Read the model definition and answer for the solid it produces. Units are mm, in the model's axes. A direction names the side the tool comes from. Give positions to 0.01 mm unless a question says otherwise; leave off trailing zeros. Write each loop counter-clockwise with the first axis right and the second up, starting at its lowest first coordinate (ties: lowest second). Pieces come first, ordered by that corner, then holes. Notation, with made-up numbers: M -18.5,57.25 L 35.5,57.25 A24 ccw 35.5,87.25 Z; hole C 42.5,-8 d5. An arc over 180 degrees is marked long. Answer as CSV lines item,"result". Start each with the question number.
```python
from build123d import *

# Parameters (mm, degrees)
T_LE_DE_BASE_PLI_E1_DEPTH             = 20.5
ESQUISSE8_W                           = 24
ESQUISSE8_H                           = 2
BOSS_EXTRU_1_DEPTH                    = 8.5
T_LE_PLI_E_SUR_AR_TE1_STRIP_W         = 10
T_LE_PLI_E_SUR_AR_TE1_STRIP_H         = 2
T_LE_PLI_E_SUR_AR_TE1_STRIP_CUT_DEPTH = 8.5
T_LE_PLI_E_SUR_AR_TE1_DEPTH           = 8.5
ESQUISSE12_W                          = 1.5
ESQUISSE12_H                          = 12
ENL_V_MAT_EXTRU_1_DEPTH               = 8.5
DIAM_TRE_DU_PER_AGE_4_0_4_1_D         = 4
DIAM_TRE_DU_PER_AGE_8_0_8_1_D         = 8
F_3_0_3_DIAMETER_HOLE3_D              = 3
R_P_TITION_CIRCULAIRE1_COUNT          = 4
DIAM_TRE_DU_PER_AGE_4_0_4_2_D         = 4
F_3_0_3_DIAMETER_HOLE1_D              = 3
CIRPATTERN1_COUNT                     = 4
CONG_1_R                              = 4
DIAM_TRE_DU_PER_AGE_8_0_8_2_D         = 8
F_3_0_3_DIAMETER_HOLE2_D              = 3
R_P_TITION_CIRCULAIRE2_COUNT          = 4


# Sheet-metal steps are written as plain solids
with BuildPart() as part:
    # Esquisse1 → Tôle de base pliée1 (new body)
    with BuildSketch(Plane(origin=(0, 0, 0), x_dir=(0, 0, -1), z_dir=(1, 0, 0))):
        with BuildLine():
            Line((0, 27), (0, 3))
            ThreePointArc((0, 3), (-0.878679656, 0.878679656), (-3, 0))
            Line((-3, 0), (-37.5, 0))
            Line((-37.5, 0), (-37.5, 2))
            Line((-37.5, 2), (-3, 2))
            ThreePointArc((-3, 2), (-2.292893219, 2.292893219), (-2, 3))
            Line((-2, 3), (-2, 27))
            Line((-2, 27), (0, 27))
        make_face()
    extrude(amount=T_LE_DE_BASE_PLI_E1_DEPTH)

    # Esquisse8 → Boss.-Extru.1 (add)
    with BuildSketch(Plane(origin=(20.5, 0, 0), x_dir=(0, 0, -1), z_dir=(1, 0, 0))):
        with Locations((-19, 1)):
            Rectangle(ESQUISSE8_W, ESQUISSE8_H)
    extrude(amount=BOSS_EXTRU_1_DEPTH)

    # Tôle pliée sur arête1 strip (across the edge) → Tôle pliée sur arête1 strip cut (cut)
    with BuildSketch(Plane(origin=(20.5, 2, 31), x_dir=(0, 0, -1), z_dir=(1, 0, 0))):
        with Locations((-4, -1)):
            Rectangle(T_LE_PLI_E_SUR_AR_TE1_STRIP_W, T_LE_PLI_E_SUR_AR_TE1_STRIP_H)
    extrude(amount=T_LE_PLI_E_SUR_AR_TE1_STRIP_CUT_DEPTH, mode=Mode.SUBTRACT)

    # Tôle pliée sur arête1 section (across the edge) → Tôle pliée sur arête1 (add)
    with BuildSketch(Plane(origin=(20.5, 2, 31), x_dir=(0, 0, -1), z_dir=(1, 0, 0))):
        with BuildLine():
            Line((-2, 1), (-2, 25))
            Line((-2, 25), (0, 25))
            Line((0, 25), (0, 1))
            ThreePointArc((0, 1), (0.292893219, 0.292893219), (1, 0))
            Line((1, 0), (1, -2))
            ThreePointArc((1, -2), (-1.121320344, -1.121320344), (-2, 1))
        make_face()
    extrude(amount=T_LE_PLI_E_SUR_AR_TE1_DEPTH)

    # Esquisse12 → Enlèv. mat.-Extru.1 (cut)
    with BuildSketch(Plane(origin=(0, 2, 0), x_dir=(1, 0, 0), z_dir=(0, 1, 0))):
        with Locations((19.75, -31.5)):
            Rectangle(ESQUISSE12_W, ESQUISSE12_H)
    extrude(amount=-ENL_V_MAT_EXTRU_1_DEPTH, mode=Mode.SUBTRACT)

    # Diamètre du perçage Ø4.0 (4)1 (through all)
    with Locations(Plane(origin=(0, 2, 0), x_dir=(1, 0, 0), z_dir=(0, 1, 0))):
        with Locations((24.25, -12.13), (24.25, -22.13)):
            Hole(DIAM_TRE_DU_PER_AGE_4_0_4_1_D / 2)

    # Diamètre du perçage Ø8.0 (8)1 (through all)
    with Locations(Plane(origin=(0, 2, 0), x_dir=(1, 0, 0), z_dir=(0, 1, 0))):
        with Locations((10.75, -22.63)):
            Hole(DIAM_TRE_DU_PER_AGE_8_0_8_1_D / 2)

    # Ø3.0 (3) Diameter Hole3 (through all)
    with Locations(Plane(origin=(0, 2, 0), x_dir=(1, 0, 0), z_dir=(0, 1, 0))):
        with Locations((10.75, -15.63)):
            f_3_0_3_diameter_hole3 = Hole(F_3_0_3_DIAMETER_HOLE3_D / 2)

    # Répétition circulaire1: Ø3.0 (3) Diameter Hole3 ×4 about axis
    r_p_tition_circulaire1_axis = Axis((10.75, 0, 22.63), (0, 1, 0))
    for i in range(1, R_P_TITION_CIRCULAIRE1_COUNT):
        add(f_3_0_3_diameter_hole3.rotate(r_p_tition_circulaire1_axis, i * 360 / R_P_TITION_CIRCULAIRE1_COUNT), mode=Mode.SUBTRACT)

    # Diamètre du perçage Ø4.0 (4)2 (through all)
    with Locations(Plane.XY.offset(33)):
        with Locations((24.25, 19.87), (24.25, 9.87)):
            Hole(DIAM_TRE_DU_PER_AGE_4_0_4_2_D / 2)

    # Ø3.0 (3) Diameter Hole1 (through all)
    with Locations(Plane.XY.offset(2)):
        with Locations((11, 14.87), (11, 21.87)):
            f_3_0_3_diameter_hole1 = Hole(F_3_0_3_DIAMETER_HOLE1_D / 2)

    # CirPattern1: Ø3.0 (3) Diameter Hole1 ×4 about axis
    cirpattern1_axis = Axis((11, 14.87, 0), (0, 0, 1))
    for i in range(1, CIRPATTERN1_COUNT):
        add(f_3_0_3_diameter_hole1.rotate(cirpattern1_axis, i * 360 / CIRPATTERN1_COUNT), mode=Mode.SUBTRACT)

    # Congé1
    cong_1_edges = [part.edges().sort_by_distance(p)[0] for p in [
        (20.5, 27, 1),
        (29, 1, 7),
        (29, 27, 32),
        (19, 1, 37.5),
    ]]
    fillet(cong_1_edges, radius=CONG_1_R)

    # Symétrie1: part across plane


with BuildPart() as part_1:
    add(part.part)
    add(part.part.mirror(Plane(origin=(0, 3, 3), x_dir=(0, 0, 1), z_dir=(1, 0, 0))))

    # Diamètre du perçage Ø8.0 (8)2 (through all)
    with Locations(Plane(origin=(0, 2, 0), x_dir=(1, 0, 0), z_dir=(0, 1, 0))):
        with Locations((0, -12.13)):
            Hole(DIAM_TRE_DU_PER_AGE_8_0_8_2_D / 2)

    # Ø3.0 (3) Diameter Hole2 (through all)
    with Locations(Plane(origin=(0, 2, 0), x_dir=(1, 0, 0), z_dir=(0, 1, 0))):
        with Locations((0, -5.13)):
            f_3_0_3_diameter_hole2 = Hole(F_3_0_3_DIAMETER_HOLE2_D / 2)

    # Répétition circulaire2: Ø3.0 (3) Diameter Hole2 ×4 about axis
    r_p_tition_circulaire2_axis = Axis((0, 0, 12.13), (0, 1, 0))
    for i in range(1, R_P_TITION_CIRCULAIRE2_COUNT):
        add(f_3_0_3_diameter_hole2.rotate(r_p_tition_circulaire2_axis, i * 360 / R_P_TITION_CIRCULAIRE2_COUNT), mode=Mode.SUBTRACT)


solid = part_1.part
```
1. Find section C-C on x = 10.75. State how many separate pieces and enclosed holes the cut face has, then the cut area to 3 significant figures.
2. Find section B-B on x = -14. Determine the outline of the cut face in (y, z), then the cut area to 3 significant figures.
3. Determine the mould class of faces 5 (the face through (0, 27, 1)), 6 (the face through (-20, 1, 25.5)), 7 (the face through (27.797, 25.859, 31.986)), 8 (the face through (-26.248, 0.986, 22.042)) for opening direction X: +X half, -X half, draft (parallel to the pull), parting line (faces both ways), or undercut.
4. Find section A-A on z = 12.13. Determine the outline of the cut face in (x, y).
5. For faces 1 (the face through (20, 1, 25.5)), 2 (the face through (11.195, 16.357, 0.986)), 3 (the face through (-24.69, 0.86, 32.1)), 4 (the face through (23, 1, 7)), determine the directions among +Z, -Z, +X, -X, +Y, -Y from which every point of the face is accessible in a straight line to the end or side of a thin tool.
6. Given pin 1 (4 mm diameter, centred on x = 5, z = 11.5, fed in from +Y); pin 2 (1.5 mm diameter, centred on x = 6.5, y = 6.5, fed in from -Z); pin 3 (6.5 mm diameter, centred on x = -24.25, y = 19.87, fed in from +Z); pin 4 (7.5 mm diameter, centred on y = 12, z = 2, fed in from +X), each flat-ended and moving along its own axis, determine where each tip first touches the part or whether it passes through.
7. Find the intervals of material crossed by line 1 (Z direction, x = 10.75, y = 0.95); line 2 (Z direction, x = 24.25, y = 1.2); line 3 (Y direction, x = 24, z = 32), in increasing order. Write a range as [from, to].
Computed:
1,separate pieces,"7"
1,enclosed holes,"0"
1,area,"77.5 mm^2"
2,outline,"M 0,3 A3 ccw 3,0 L 27,0 L 27,2 L 3,2 A1 cw 2,3 L 2,20.3 L 0,20.3 Z; M 0,24.96 L 2,24.96 L 2,37.5 L 0,37.5 Z"
2,area,"114 mm^2"
3,face 5,"draft"
3,face 6,"undercut"
3,face 7,"+X half"
3,face 8,"undercut"
4,outline,"M -29,0 L -26.25,0 L -26.25,2 L -29,2 Z; M -22.25,0 L -8.5,0 L -8.5,2 L -22.25,2 Z; M -5.5,0 L -4,0 L -4,2 L -5.5,2 Z; M 4,0 L 5.5,0 L 5.5,2 L 4,2 Z; M 8.5,0 L 22.25,0 L 22.25,2 L 8.5,2 Z; M 26.25,0 L 29,0 L 29,2 L 26.25,2 Z"
5,face 1,"+Z, +Y, -Y"
5,face 2,"+Z, -Z"
5,face 3,"+Z, -X, -Y"
5,face 4,"-Z, +X, +Y, -Y"
6,pin 1,"stops at y = 2"
6,pin 2,"stops at z = 0"
6,pin 3,"stops at z = 33"
6,pin 4,"stops at x = 20.5"
7,line 1,"z = [0.81, 14.13], [17.13, 18.63], [26.63, 28.13], [31.13, 37.5]"
7,line 2,"z = [7, 10.13], [14.13, 20.13], [24.13, 32.4]"
7,line 3,"y = [0.76, 7.89], [11.85, 17.89], [21.85, 27]"
